Geometry check sheet. Reference: the model listing, model coordinates, mm. A direction names the side the tool comes from. Round coordinates to 2 decimals unless told otherwise and drop trailing zeros. Order: outer loops, then holes, each group sorted by start corner. A loop starts at its lowest first (then second) coordinate and runs counter-clockwise, first axis right, second up.
(1) Cross-section at B-B on x = 71.5. Enter the section's corners in (y, z).
(2) Thickness scan on L1, parallel to X at y = 4.5, z = -4 (3 decimals); L2, parallel to X at y = -28.5, z = -5.25 (3 decimals); L3, parallel to Y at x = 26.5, z = -6.5. Record the ranges inside material, lowest first.
(3) Cross-section at A-A on y = -26. Enter the section's corners in (x, z) (3 decimals).
(4) Cross-section at C-C on x = 0. Enter the section's corners in (y, z).
(5) Draft check along Y on faces 4 (the face through (47.96, -1.97, -0.76)), 5 (the face through (112, -6, 0)). Enter one of: pulls with the +Y half, pulls with the -Y half, needs draft (parallel to the pull), parting line crosses it, or undercut.
(6) Set-up check for faces 1 (the face through (40.97, -53.87, -0.76)), 2 (the face through (38.145, -20, -5)), 3 (the face through (-5.07, -19, -5)): record each of +Z, -Z, +X, -X, +Y, -Y from which the full face is reachable in a straight line by a thin tool's end or side.
(7) Gauge pin test, flat ends, axial feed: P1, Ø1.2, axis at x = 18.5, z = -4, coming from the -Y side; P2, Ø3, axis at y = -14.5, z = -5.5, coming from the -X side; P3, Ø4, axis at x = 7.5, z = -4, coming from the +Y side. Record the tip position at first contact, or that the pin passes through.
from build123d import *

# Parameters (mm, degrees)
SKETCH_R      = 1.5
SKETCH_R_2    = 3
SKETCH_W      = 33.214997
SKETCH_H      = 76.52
SKETCH_W_2    = 30.035003
SKETCH_W_3    = 10.005
SKETCH_H_2    = 21.910002
PAD_DEPTH     = 4
SKETCH001_R   = 4
SKETCH001_R_2 = 1.5
PAD001_DEPTH  = 3
FILLET_R      = 1.5
SKETCH002_W   = 10
SKETCH002_H   = 1
POCKET_DEPTH  = 2
CHAMFER_SIZE  = 1.5


with BuildPart() as obj1:
    # Sketch → Pad (new body)
    with BuildSketch(Plane.XY):
        with BuildLine():
            ThreePointArc((2.930002, 28.879999), (-10.726853, 34.536854), (-5.069998, 20.879999))
            Line((-5.069998, 20.879999), (-5.069998, -59.640001))
            ThreePointArc((-5.069998, -59.640001), (-10.726853, -73.296855), (2.930002, -67.640001))
            Line((2.930002, -67.640001), (82.180002, -67.640001))
            ThreePointArc((82.180002, -67.640001), (95.836856, -73.296855), (90.180002, -59.640001))
            Line((90.180002, -48.259999), (90.180002, -59.640001))
            Line((104.184999, -48.259999), (90.180002, -48.259999))
            ThreePointArc((104.184999, -48.259999), (114.427638, -52.502641), (110.185002, -42.259999))
            Line((110.185002, -12.349997), (110.185002, -42.259999))
            ThreePointArc((110.185002, -12.349997), (114.427643, -2.107356), (104.185002, -6.349997))
            Line((90.180002, -6.349997), (104.185002, -6.349997))
            Line((90.180002, 20.879999), (90.180002, -6.349997))
            ThreePointArc((90.180002, 20.879999), (95.836856, 34.536854), (82.180002, 28.879999))
            Line((2.930002, 28.879999), (82.180002, 28.879999))
        make_face()
        with Locations((44.145001, -51.434998)):
            Circle(SKETCH_R, mode=Mode.SUBTRACT)
        with Locations((110.184999, -48.259999)):
            Circle(SKETCH_R, mode=Mode.SUBTRACT)
        with Locations((44.144999, -3.174998)):
            Circle(SKETCH_R, mode=Mode.SUBTRACT)
        with Locations((110.185002, -6.349997)):
            Circle(SKETCH_R, mode=Mode.SUBTRACT)
        with Locations((-5.069998, 28.879999)):
            Circle(SKETCH_R_2, mode=Mode.SUBTRACT)
        with Locations((-5.069998, -67.640001)):
            Circle(SKETCH_R_2, mode=Mode.SUBTRACT)
        with Locations((90.180002, -67.640001)):
            Circle(SKETCH_R_2, mode=Mode.SUBTRACT)
        with Locations((90.180002, 28.879999)):
            Circle(SKETCH_R_2, mode=Mode.SUBTRACT)
        with Locations((21.537501, -19.380001)):
            Rectangle(SKETCH_W, SKETCH_H, mode=Mode.SUBTRACT)
        with Locations((65.1625, -19.380001)):
            Rectangle(SKETCH_W_2, SKETCH_H, mode=Mode.SUBTRACT)
        with Locations((95.182502, -27.304998)):
            Rectangle(SKETCH_W_3, SKETCH_H_2, mode=Mode.SUBTRACT)
    extrude(amount=PAD_DEPTH)


with BuildPart() as top_supports_final:
    # Pad001 base: copy of obj1
    add(obj1.part)

    # Sketch001 → Pad001 (new body)
    with BuildSketch(Plane.XY.offset(4)):
        with Locations((44.144999, -3.174998)):
            Circle(SKETCH001_R)
        with Locations((44.144999, -3.174998)):
            Circle(SKETCH001_R_2, mode=Mode.SUBTRACT)
        with Locations((44.145001, -51.434998)):
            Circle(SKETCH001_R)
        with Locations((44.145001, -51.434998)):
            Circle(SKETCH001_R_2, mode=Mode.SUBTRACT)
        with Locations((110.184999, -48.259999)):
            Circle(SKETCH001_R)
        with Locations((110.184999, -48.259999)):
            Circle(SKETCH001_R_2, mode=Mode.SUBTRACT)
        with Locations((110.185002, -6.349997)):
            Circle(SKETCH001_R)
        with Locations((110.185002, -6.349997)):
            Circle(SKETCH001_R_2, mode=Mode.SUBTRACT)
    extrude(amount=PAD001_DEPTH)


with BuildPart() as top_support_fillets:
    # Fillet base: copy of top_supports_final
    add(top_supports_final.part)

    # Fillet
    fillet_edges = [top_support_fillets.edges().sort_by_distance(p)[0] for p in [
        (106.184999, -48.259999, 4),
        (40.144999, -3.174998, 4),
        (40.145001, -51.434998, 4),
        (106.185002, -6.349997, 4),
    ]]
    fillet(fillet_edges, radius=FILLET_R)


with BuildPart() as base_rough:
    # Fusion base: copy of obj1
    add(obj1.part)

    # Fusion: union top_support_fillets, top_supports_final
    add(top_support_fillets.part)
    add(top_supports_final.part)


with BuildPart() as base_rough_1:
    # Fusion placement: moved
    add(base_rough.part.moved(Location((0, 0, -7))))


with BuildPart() as hdmi_clearance:
    # Pocket base: copy of base_rough
    add(base_rough_1.part)

    # Sketch002 → Pocket (cut)
    with BuildSketch(Plane(origin=(110.185002, 0, -7), x_dir=(0, 1, 0), z_dir=(1, 0, 0))):
        with Locations((-29.259999, 3.5)):
            Rectangle(SKETCH002_W, SKETCH002_H)
    extrude(amount=-POCKET_DEPTH, mode=Mode.SUBTRACT)


with BuildPart() as chamfer_body:
    # Chamfer base: copy of base_rough
    add(base_rough_1.part)

    # Chamfer
    chamfer_edges = [chamfer_body.edges().sort_by_distance(p)[0] for p in [
        (42.644999, -3.174998, -7),
        (42.645001, -51.434998, -7),
        (108.684999, -48.259999, -7),
        (108.685002, -6.349997, -7),
    ]]
    chamfer(chamfer_edges, length=CHAMFER_SIZE)


with BuildPart() as obj2:
    # Common base: copy of base_rough
    add(base_rough_1.part)

    # Common: intersect hdmi_clearance, Chamfer body
    add(hdmi_clearance.part, mode=Mode.INTERSECT)
    add(chamfer_body.part, mode=Mode.INTERSECT)


solid = obj2.part
Found:
1. outline: (-67.64, -7) - (-57.64, -7) - (-57.64, -3) - (-67.64, -3) - close; (18.88, -7) - (28.88, -7) - (28.88, -3) - (18.88, -3) - close
2. L1: x = -5.07 to 4.93, 38.145 to 50.145, 80.18 to 90.18
2. L2: x = -5.07 to 4.93, 38.145 to 50.145, 80.18 to 90.18, 100.185 to 110.185
2. L3: y = -67.64 to -57.64, 18.88 to 28.88
3. outline: (-5.07, -7) - (4.93, -7) - (4.93, -3) - (-5.07, -3) - close; (38.145, -7) - (50.145, -7) - (50.145, -3) - (38.145, -3) - close; (80.18, -7) - (90.18, -7) - (90.18, -3) - (80.18, -3) - close; (100.185, -7) - (110.185, -7) - (110.185, -4) - (108.185, -4) - (108.185, -3) - (100.185, -3) - close
4. outline: (-73.83, -7) - (35.07, -7) - (35.07, -3) - (-73.83, -3) - close
5. face 4: undercut
5. face 5: needs draft
6. face 1: +Z
6. face 2: +Z, -Z
6. face 3: +Z, -Z, -X
7. P1: stops at y = -67.64
7. P2: stops at x = -5.07
7. P3: stops at y = 28.88
